from build123d import *

# Parameters (mm, degrees)
F0_R     = 10
F0_W     = 40
F0_H     = 40
F1_DEPTH = 6


with BuildPart() as f1:
    # F0 (on Front) → F1 (new body)
    with BuildSketch(Plane.XZ):
        Polygon((20.309229, -90.934532), (63.055574, -68.597), (88.906229, -27.878958), (90.934532, 20.309229), (68.597, 63.055574), (27.878958, 88.906229), (-20.309229, 90.934532), (-63.055574, 68.597), (-88.906229, 27.878958), (-90.934532, -20.309229), (-68.597, -63.055574), (-27.878958, -88.906229), align=None)
        with Locations((-42.426407, -42.426407)):
            Circle(F0_R, mode=Mode.SUBTRACT)
        with Locations((0, -60)):
            Circle(F0_R, mode=Mode.SUBTRACT)
        with Locations((42.426407, -42.426407)):
            Circle(F0_R, mode=Mode.SUBTRACT)
        with Locations((-60, 0)):
            Circle(F0_R, mode=Mode.SUBTRACT)
        with Locations((-42.426407, 42.426407)):
            Circle(F0_R, mode=Mode.SUBTRACT)
        Rectangle(F0_W, F0_H, mode=Mode.SUBTRACT)
        with Locations((42.426407, 42.426407)):
            Circle(F0_R, mode=Mode.SUBTRACT)
        with Locations((60, 0)):
            Circle(F0_R, mode=Mode.SUBTRACT)
        with Locations((0, 60)):
            Circle(F0_R, mode=Mode.SUBTRACT)
    extrude(amount=F1_DEPTH)


solid = f1.part
Check sheet for the modelled part. Datum: model origin and axes. Units: mm. A direction names the side the tool comes from. Round coordinates to 2 decimals unless told otherwise and drop trailing zeros. Order: outer loops, then holes, each group sorted by start corner. A loop starts at its lowest first (then second) coordinate and runs counter-clockwise, first axis right, second up.
(1) Go/stop test with flat-tipped pins: P1, Ø16, axis at x = 0, z = -60, coming from the +Y side; P2, Ø2, axis at y = -4.5, z = -3.5, coming from the +X side; P3, Ø2, axis at y = -1, z = -17, coming from the +X side; P4, Ø2, axis at x = -67.5, y = -1, coming from the -Z side. Record where each tip stops, or that it passes through.
(2) Scan lines: probe 1 along Z at (x, y) = (7, -0.3); probe 2 along X at (y, z) = (-5.6, 7); probe 3 along Z at (x, y) = (-36, -1.9). Record each from-to range of solid material in increasing order.
(3) Cross-section at A-A, the plane z = 0. Enter the section's corners in (x, y).
(4) Access from +Z, -Z, +X, -X, +Y, -Y to the whole of each face (thin tool, end or side, straight path). Record for faces 5 (the flat face through (79.922, -2.958, 41.383)), 6 (the flat face through (-20, -3, 0)).
(5) Cross-section at C-C, the plane x = 66.5. Enter the section's corners in (y, z), and give its area (3 significant figures).
(6) Cross-section at B-B, the plane x = 35. Enter the section's corners in (y, z).
(7) Cross-section at D-D, the plane z = -57. Enter the section's corners in (x, y), and give its area (3 significant figures).
(8) Draft check along X on faces 1 (the flat face through (-1, 0, 21)), 2 (the cylindrical face through (-2.17, -2.96, 50.24)), 3 (the flat face through (89.906, -2.958, -4.122)), 4 (the flat face through (-79.922, -2.958, -41.383)). Enter one of: pulls with the +X half, pulls with the -X half, needs draft (parallel to the pull), parting line crosses it, or undercut.
Check sheet entries:
1. P1: passes through
1. P2: stops at x = 89.97
1. P3: stops at x = 89.41
1. P4: stops at z = -64.39
2. probe 1: z = -90.37 to -67.14, -52.86 to -20, 20 to 52.86, 67.14 to 89.79
2. probe 2: x = -89.79 to -67.14, -52.86 to -20, 20 to 52.86, 67.14 to 90.37
2. probe 3: z = -83.75 to -50.09, -34.76 to 34.76, 50.09 to 82.74
3. outline: (-90.08, -6) - (-70, -6) - (-70, 0) - (-90.08, 0) - close; (-50, -6) - (-20, -6) - (-20, 0) - (-50, 0) - close; (20, -6) - (50, -6) - (50, 0) - (20, 0) - close; (70, -6) - (90.08, -6) - (90.08, 0) - (70, 0) - close
4. face 5: +Z, +X, +Y, -Y
4. face 6: +Y, -Y
5. outline: (-6, -63.17) - (0, -63.17) - (0, -7.6) - (-6, -7.6) - close; (-6, 7.6) - (0, 7.6) - (0, 64.39) - (-6, 64.39) - close
5. area: 674 mm2
6. outline: (-6, -83.26) - (0, -83.26) - (0, -49.12) - (-6, -49.12) - close; (-6, -35.73) - (0, -35.73) - (0, 35.73) - (-6, 35.73) - close; (-6, 49.12) - (0, 49.12) - (0, 84.39) - (-6, 84.39) - close
7. outline: (-71.76, -6) - (-9.54, -6) - (-9.54, 0) - (-71.76, 0) - close; (9.54, -6) - (70.42, -6) - (70.42, 0) - (9.54, 0) - close
7. area: 739 mm2
8. face 1: needs draft
8. face 2: undercut
8. face 3: pulls with the +X half
8. face 4: pulls with the -X half
